Can you work these out from the model? Positions are in its coordinate system, mm. A direction names the side the tool comes from. Round coordinates to 2 decimals unless told otherwise and drop trailing zeros. Order: outer loops, then holes, each group sorted by start corner. A loop starts at its lowest first (then second) coordinate and runs counter-clockwise, first axis right, second up. Notation, with made-up numbers: (76, 61) - (129, 61) arc R11 cw to (129, 71) - close; hole circle Ø3 at (36, 6.25). An arc over 180 degrees is marked (long way). Write item = value, one per line.
from build123d import *

# Parameters (mm, degrees)
F0_W      = 48
F0_H      = 40
F1_DEPTH  = 4
F2_R      = 2
F3_DEPTH  = 4.001
F4_W      = 29.5
F4_H      = 15
F5_DEPTH  = 12.5
F6_W      = 15
F6_H      = 0.034775
F6_H_2    = 3.5
F7_DEPTH  = 1.6
F8_W      = 15
F8_H      = 3.5
F9_DEPTH  = 1.6
F10_DEPTH = 1.6
F11_W     = 33.5
F11_H     = 7
F12_DEPTH = 2


with BuildPart() as f1:
    # F0 (on Top) → F1 (new body)
    with BuildSketch(Plane.XY):
        Rectangle(F0_W, F0_H)
    extrude(amount=F1_DEPTH)

    # F2 (on face) → F3 (cut, through all)
    with BuildSketch(Plane.XY.offset(4)):
        with Locations((-14.224, 14.224)):
            Circle(F2_R)
        with Locations((14.224, 14.224)):
            Circle(F2_R)
        with Locations((-14.224, -14.224)):
            Circle(F2_R)
        with Locations((14.224, -14.224)):
            Circle(F2_R)
    extrude(amount=-F3_DEPTH, mode=Mode.SUBTRACT)

    # F4 (on face) → F5 (join)
    with BuildSketch(Plane.XY.offset(4)):
        Rectangle(F4_W, F4_H)
    extrude(amount=F5_DEPTH)

    # F6 (on face) → F7 (cut)
    with BuildSketch(Plane(origin=(-14.75, 0, 0), x_dir=(0, -1, 0), z_dir=(-1, 0, 0))):
        with Locations((0, 3.982613)):
            Rectangle(F6_W, F6_H)
        with Locations((0, 5.75)):
            Rectangle(F6_W, F6_H_2)
    extrude(amount=-F7_DEPTH, mode=Mode.SUBTRACT)

    # F8 (on face) → F9 (cut)
    with BuildSketch(Plane.YZ.offset(14.75)):
        with Locations((0, 5.75)):
            Rectangle(F8_W, F8_H)
    extrude(amount=-F9_DEPTH, mode=Mode.SUBTRACT)

    # F6 (on face) → F10 (cut)
    with BuildSketch(Plane(origin=(-14.75, 0, 0), x_dir=(0, -1, 0), z_dir=(-1, 0, 0))):
        with Locations((0, 3.982613)):
            Rectangle(F6_W, F6_H)
        with Locations((0, 5.75)):
            Rectangle(F6_W, F6_H_2)
    extrude(amount=-F10_DEPTH, mode=Mode.SUBTRACT)

    # F11 (on face) → F12 (join)
    with BuildSketch(Plane.XZ.offset(7.5)):
        with Locations((0, 7.5)):
            Rectangle(F11_W, F11_H)
    extrude(amount=F12_DEPTH)


solid = f1.part
(1) If we section it at A-A (z = 10): Write out the boundary of the cut face in (x, y), plus the area to 4 significant figures.
Computed:
outline = (-16.75, -9.5) - (16.75, -9.5) - (16.75, -7.5) - (14.75, -7.5) - (14.75, 7.5) - (-14.75, 7.5) - (-14.75, -7.5) - (-16.75, -7.5) - close
area = 509.5 mm^2
(2) If we section it at B-B (y = 13.5): Write out the boundary of the cut face in (x, z).
Computed:
outline = (-24, 0) - (-16.09, 0) - (-16.09, 4) - (-24, 4) - close; (-12.36, 0) - (12.36, 0) - (12.36, 4) - (-12.36, 4) - close; (16.09, 0) - (24, 0) - (24, 4) - (16.09, 4) - close
(3) On a 3-axis mill with a long thin cutter (end or side, diameter ignored), from which of +Z, -Z, +X, -X, +Y, -Y can I reach the whole of each face in a straight line? I mean faces 5 (the face through (16.75, -8, 7)), 6 (the face through (13.15, 0, 6)), 7 (the face through (14.75, 0, 12)), 8 (the face through (0, -7.5, 14)). Say none if no direction works.
Computed:
face_5 = +Z, +X, +Y, -Y
face_6 = +X, +Y
face_7 = +Z, +X, +Y
face_8 = +Z, +X, -X, -Y
(4) Thinking about a two-plate mould opening in Z: for faces 1 (the face through (-14, 0, 3.965)), 2 (the face through (0, -9.5, 8)), 3 (the face through (-14, 0, 7.5)), 4 (the face through (0, -8, 11)), which applies, +Z half, -Z half, draft (parallel to the pull), parting line (faces both ways), or undercut?
Computed:
face_1 = undercut
face_2 = draft
face_3 = undercut
face_4 = +Z half
(5) If I drill on line 1 (Y direction, x = 15, z = 1.25); line 2 (X direction, y = -13, z = 2.75); line 3 (Z direction, x = -1.5, y = -12.5), over which ranges is the centre line in solid material (lowest first)? Write a range as from..to.
Computed:
line_1 = -20..-16.07, -12.38..12.38, 16.07..20
line_2 = -24..-15.81, -12.64..12.64, 15.81..24
line_3 = 0..4
(6) If we section it at C-C (z = 2): Write out the boundary of the cut face in (x, y).
Computed:
outline = (-24, -20) - (24, -20) - (24, 20) - (-24, 20) - close; hole circle Ø4 at (-14.22, -14.22); hole circle Ø4 at (-14.22, 14.22); hole circle Ø4 at (14.22, -14.22); hole circle Ø4 at (14.22, 14.22)
(7) Will these pins go through, and if not, where does the flat tip stop? P1, Ø8, axis at y = -5.5, z = 9, coming from the -X side; P2, Ø4.5, axis at x = -2, z = 13.5, coming from the -Y side; P3, Ø5, axis at x = 16.5, y = 12.5, coming from the +Z side.
Computed:
P1 = -16.75
P2 = -7.5
P3 = 4
(8) If we section it at D-D (x = 10.5): Write out the boundary of the cut face in (y, z), plus the area to 4 significant figures.
Computed:
outline = (-20, 0) - (20, 0) - (20, 4) - (7.5, 4) - (7.5, 16.5) - (-7.5, 16.5) - (-7.5, 11) - (-9.5, 11) - (-9.5, 4) - (-20, 4) - close
area = 361.5 mm^2
